CAD build for the part. Positions are in the model's coordinates, mm. Round coordinates to 2 decimals unless told otherwise and drop trailing zeros. Loops run counter-clockwise (first coordinate to the right, second up) from the corner with the lowest first, then second, coordinate; pieces in that order, holes last. Notation, with made-up numbers: M 82.5,17 L 127.5,17 A38 cw 127.5,55 Z; hole C -39.5,11 d10. An arc over 180 degrees is marked long. Use a Markdown table: item, result. Add a question column.
(1) Flat gauge pins, fed straight in: P1, Ø0.5, axis at x = 317, z = -7, coming from the +Y side; P2, Ø19, axis at x = 146.5, y = 17.5, coming from the +Z side; P3, Ø0.8, axis at x = 166.5, z = -7, coming from the -Y side. Where does each tip first touch, or does it go through?
(2) Band-saw the part on A-A, the plane y = 9. Write the cut outline in (x, z).
(3) Wall check: L1, parallel to Y at x = 156.5, z = -3.25; L2, parallel to Y at x = 355.5, z = -1.25; L3, parallel to Z at x = 326.5, y = 21. Give the ranges that are in metal, low to high.
Autodesk Inventor part; units mm, degrees
ref_plane "YZ Plane" through (0, 0, 0) normal (1, 0, 0) x (0, 1, 0)
ref_plane "XZ Plane" through (0, 0, 0) normal (0, 1, 0) x (-1, 0, 0)
ref_plane "XY Plane" through (0, 0, 0) normal (0, 0, 1) x (1, 0, 0)
sketch "Boceto principal" plane through (0, 0, 0) normal (1, 0, 0) x (0, 1, 0)
  line L0 (0, 0) -> (0, -1)
  line L1 (0, -1) -> (3.5, -1)
  line L2 (4, -1.5) -> (4, -7)
  line L3 (4.5, -7.5) -> (30.5, -7.5)
  line L4 (31, -7) -> (31, -1.5)
  line L5 (31.5, -1) -> (35, -1)
  line L6 (35, -1) -> (35, 0)
  line L7 (35, 0) -> (30.5, 0)
  line L8 (30, -0.5) -> (30, -6)
  line L9 (29.5, -6.5) -> (5.5, -6.5)
  line L10 (5, -6) -> (5, -0.5)
  line L11 (4.5, 0) -> (0, 0)
  arc A0 (4, -1.5) -> (3.5, -1) centre (3.5, -1.5) ccw
  arc A1 (4, -7) -> (4.5, -7.5) centre (4.5, -7) ccw
  arc A2 (30.5, -7.5) -> (31, -7) centre (30.5, -7) ccw
  arc A3 (31.5, -1) -> (31, -1.5) centre (31.5, -1.5) ccw
  arc A4 (30.5, 0) -> (30, -0.5) centre (30.5, -0.5) ccw
  arc A5 (29.5, -6.5) -> (30, -6) centre (29.5, -6) ccw
  arc A6 (5, -6) -> (5.5, -6.5) centre (5.5, -6) ccw
  arc A7 (5, -0.5) -> (4.5, 0) centre (4.5, -0.5) ccw
extrude "Extrusion1" add sketch "Boceto principal" along normal blind 378
sketch "Boceto agujeros" plane through (0, 0, 0) normal (0, 0, 1) x (1, 0, 0)
  line L0 (7.6, 14.9) -> (20.4, 14.9)
  line L1 (20.4, 20.1) -> (7.6, 20.1)
  arc A0 (7.6, 20.1) -> (7.6, 14.9) centre (7.6, 17.5) ccw
  arc A1 (20.4, 14.9) -> (20.4, 20.1) centre (20.4, 17.5) ccw
extrude "Extrusion2" cut sketch "Boceto agujeros" against normal blind 15
pattern_linear "Rectangular Pattern1" count 16 spacing 25 along (1, 0, 0) of "Extrusion2"
properties part number "Riel 35x7.5 378mm" material "Steel, Galvanized"
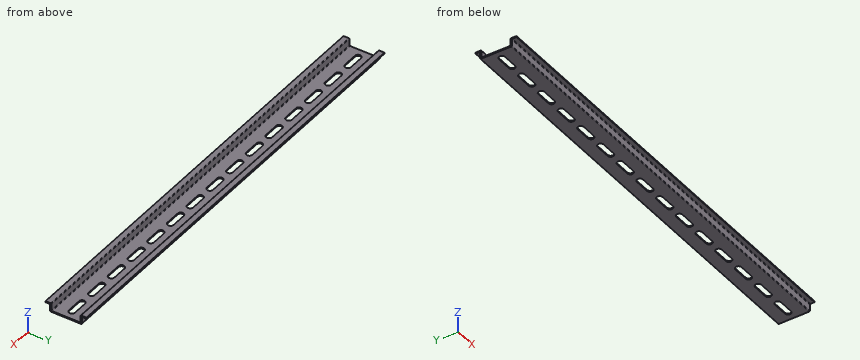
Return value:
| question | item | result |
|---|---|---|
| 1 | P1 | y = 31 |
| 1 | P2 | z = -6.5 |
| 1 | P3 | y = 4 |
| 2 | outline | M 0,-7.5 L 378,-7.5 L 378,-6.5 L 0,-6.5 Z |
| 3 | L1 | 4 to 5, 30 to 31 |
| 3 | L2 | 3.93 to 5, 30 to 31.07 |
| 3 | L3 | -7.5 to -6.5 |
